Answer from the drawing. Dimensions are ordinates in mm from the lowest x, y and z of the part. A direction names the side the tool comes from. Round coordinates to 2 decimals unless told otherwise and drop trailing zeros. Order: outer loops, then holes, each group sorted by start corner. A loop starts at its lowest first (then second) coordinate and runs counter-clockwise, first axis right, second up. Notation, with made-up numbers: (5, -1) - (16, -1) arc R26 cw to (16, 19) - close; hole circle Ø8 at (-9.75, 61.5). An arc over 180 degrees is marked (long way). One line per question, with ' | ' between items. Start each with the question number.
1) The part is cut by section B-B, the plane y = 24.5. Give the vertices of the cut face in (x, z).
2) Straight lines are drawn through the part: line 1 (Y direction, x = 22.5, z = 51.5); line 2 (Z direction, x = 39.5, y = 42.5); line 3 (Y direction, x = 16.5, z = 8) (1 decimal). For each, find the intervals that lie inside material, in ascending order. Write a range as from..to.
3) For the marked faces 1 and 2, determine the directions among +Z, -Z, +X, -X, +Y, -Y from which every point of the face is accessible in a straight line to the end or side of a thin tool.
4) The part is cut by section A-A, the plane x = 27.5. Give the vertices of the cut face in (y, z).
5) Flat-ended cylindrical pins translate along their axes: pin 1 (12 mm diameter, centred on x = 32.5, y = 25.5, fed in from -Z); pin 2 (13 mm diameter, centred on x = 29.5, y = 23.5, fed in from +Z); pin 3 (6 mm diameter, centred on x = 29.5, z = 40.5, fed in from -Y). Find the tip coordinate at first contact, or state that the pin passes through.
6) The part is cut by section D-D, the plane x = 6. Give the vertices of the cut face in (y, z) (1 decimal).
7) The part is cut by section C-C, the plane z = 31. Give the vertices of the cut face in (x, y).
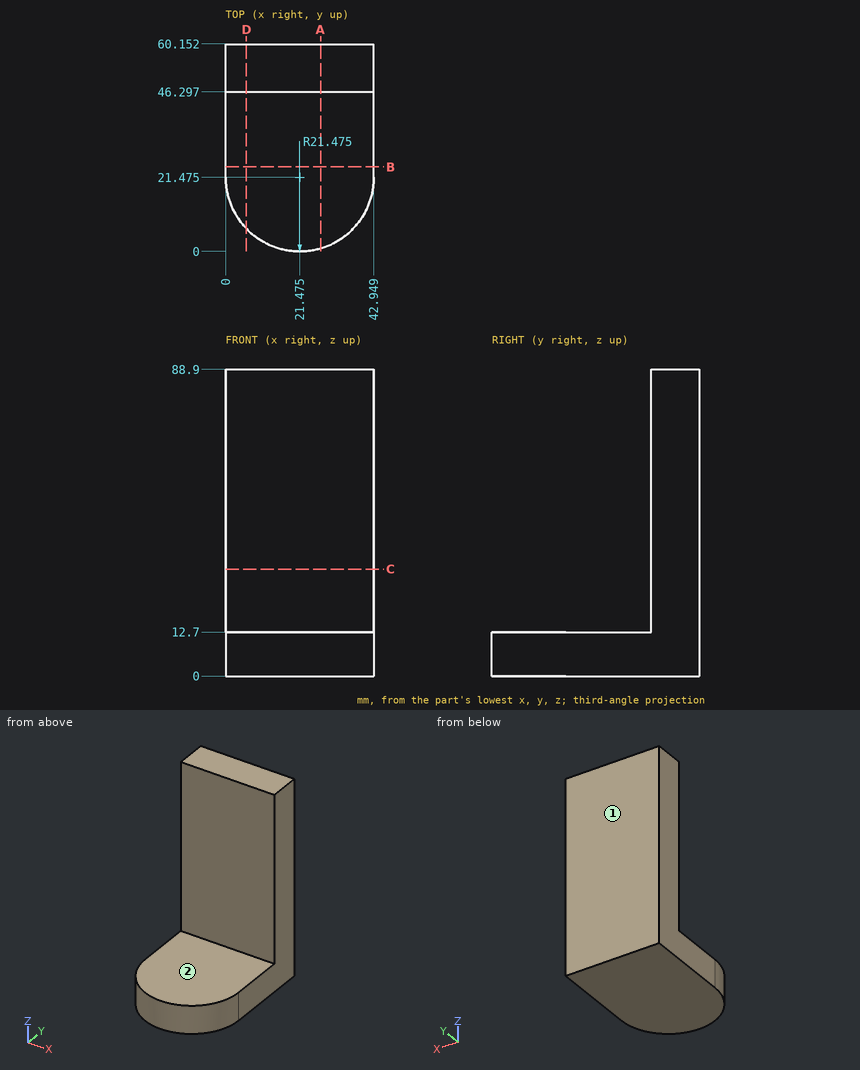
Values:
1) outline: (0, 0) - (42.95, 0) - (42.95, 12.7) - (0, 12.7) - close
2) line 1: y = 46.3..60.15 | line 2: z = 0..12.7 | line 3: y = 0.6..60.2
3) face 1: +Z, -Z, +X, -X, +Y | face 2: +Z, +X, -X, -Y
4) outline: (0.86, 0) - (60.15, 0) - (60.15, 88.9) - (46.3, 88.9) - (46.3, 12.7) - (0.86, 12.7) - close
5) pin 1: stops at z = 0 | pin 2: stops at z = 12.7 | pin 3: stops at y = 46.3
6) outline: (6.6, 0) - (60.2, 0) - (60.2, 88.9) - (46.3, 88.9) - (46.3, 12.7) - (6.6, 12.7) - close
7) outline: (0, 46.3) - (42.95, 46.3) - (42.95, 60.15) - (0, 60.15) - close
